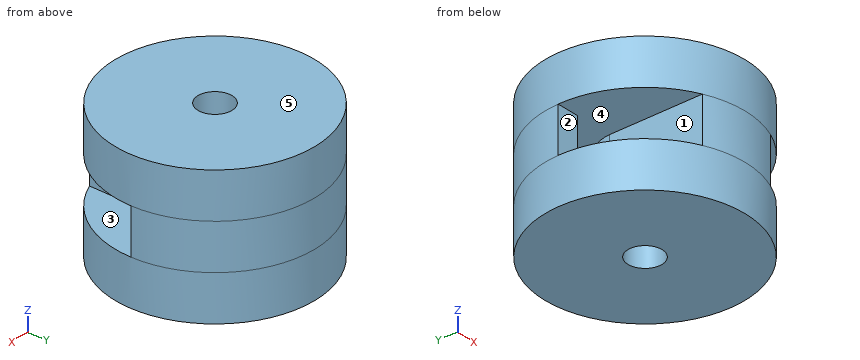
```python
from build123d import *

# Parameters (mm, degrees)
F0_R     = 11
F1_DEPTH = 5
F3_DEPTH = 5
F4_R     = 11
F5_DEPTH = 5
F6_R     = 1.875
F7_DEPTH = 25


with BuildPart() as f1:
    # F0 (on Top) → F1 (new body)
    with BuildSketch(Plane.XY):
        with Locations((-55.3302019835, -34.0237878263)):
            Circle(F0_R)
    extrude(amount=F1_DEPTH)

    # F2 (on face) → F3 (join)
    with BuildSketch(Plane.XY.offset(5)):
        with BuildLine():
            Line((-46.800726779, -33.8632795051), (-44.3313730877, -33.8632795051))
            ThreePointArc((-44.3313730877, -33.8632795051), (-55.3302019835, -23.0237878263), (-66.3290308792, -33.8632795051))
            Line((-66.3290308792, -33.8632795051), (-63.8596771879, -33.8632795051))
            ThreePointArc((-63.8596771879, -33.8632795051), (-55.3302019835, -25.9412589779), (-46.800726779, -33.8632795051))
        make_face()
        with BuildLine():
            ThreePointArc((-59.7163877129, -44.1114721367), (-55.3302019835, -45.0237878263), (-50.944016254, -44.1114721367))
            Line((-50.944016254, -44.1114721367), (-50.944016254, -34.1842961475))
            Line((-50.944016254, -34.1842961475), (-50.944016254, -33.8632795051))
            ThreePointArc((-50.944016254, -33.8632795051), (-55.3302019835, -29.6346662543), (-59.7163877129, -33.8632795051))
            Line((-59.7163877129, -33.8632795051), (-59.7163877129, -34.1842961475))
            Line((-59.7163877129, -34.1842961475), (-59.7163877129, -44.1114721367))
        make_face()
    extrude(amount=F3_DEPTH)

    # F4 (on face) → F5 (join)
    with BuildSketch(Plane.XY.offset(10)):
        with Locations((-55.3302019835, -34.0237878263)):
            Circle(F4_R)
    extrude(amount=F5_DEPTH)

    # F6 (on face) → F7 (cut)
    with BuildSketch(Plane.XY.offset(15)):
        with Locations((-55.3302019835, -34.0237878263)):
            Circle(F6_R)
    extrude(amount=-F7_DEPTH, mode=Mode.SUBTRACT)


solid = f1.part
```
Check sheet for the modelled part. Datum: model origin and axes. Units: mm. Face numbers are marked on the shaded views. A direction names the side the tool comes from. Round coordinates to 2 decimals unless told otherwise and drop trailing zeros. Order: outer loops, then holes, each group sorted by start corner. A loop starts at its lowest first (then second) coordinate and runs counter-clockwise, first axis right, second up. Notation, with made-up numbers: (39.25, -22) - (58.25, -22) arc R15 cw to (58.25, 0) - close; hole circle Ø3 at (6.5, 87.25). An arc over 180 degrees is marked (long way). Write item = value, one per line.
Q1. Go/stop test with flat-tipped pins: pin 1 (8 mm diameter, centred on x = -55.5, y = -41, fed in from -Z); pin 2 (4 mm diameter, centred on y = -41, z = 7.5, fed in from -X); pin 3 (2.5 mm diameter, centred on y = -37.5, z = 7, fed in from +X); pin 4 (5 mm diameter, centred on x = -62, z = 12, fed in from -Y). Record where each tip stops, or that it passes through.
Computed:
pin_1 = 0
pin_2 = -59.72
pin_3 = -50.94
pin_4 = -44.2
Q2. Section check A-A (y = -33). Record the boundary of the cut face in (x, z).
Computed:
outline = (-66.28, 0) - (-56.9, 0) - (-56.9, 15) - (-66.28, 15) - close; (-53.76, 0) - (-44.38, 0) - (-44.38, 15) - (-53.76, 15) - close; hole (-63.75, 5) - (-59.6, 5) - (-59.6, 10) - (-63.75, 10) - close; hole (-51.06, 5) - (-46.91, 5) - (-46.91, 10) - (-51.06, 10) - close
Q3. Section check C-C (z = 5.5). Record the boundary of the cut face in (x, y) (3 decimals), and give its area (3 significant figures).
Computed:
outline = (-66.329, -33.863) - (-63.86, -33.863) arc R8.553 cw to (-46.801, -33.863) - (-44.331, -33.863) arc R11 ccw to start; (-59.716, -44.111) arc R11 ccw to (-50.944, -44.111) - (-50.944, -33.863) arc R4.389 ccw to (-59.716, -33.863) - close; hole circle Ø3.75 at (-55.33, -34.024)
area = 196 mm^2
Q4. Thickness scan on line 1 along Z through (x, y) = (-60, -40.25); line 2 along X through (y, z) = (-33.5, 6) (3 decimals); line 3 along X through (y, z) = (-42.75, 5.5). Record the ranges inside material, lowest first.
Computed:
line_1 = 0 to 5, 10 to 15
line_2 = -66.318 to -63.825, -59.688 to -57.131, -53.53 to -50.972, -46.835 to -44.343
line_3 = -59.72 to -50.94
Q5. Tool access check on the marked faces 4 and 5. Record the directions out of +Z, -Z, +X, -X, +Y, -Y that give a thin tool (end or side, any length) a straight path to the whole face; none if there is none.
Computed:
face_4 = none
face_5 = +Z, +X, -X, +Y, -Y
Q6. Draft check along Y on the marked faces 1, 2 and 3. Enter one of: pulls with the +Y half, pulls with the -Y half, needs draft (parallel to the pull), parting line crosses it, or undercut.
Computed:
face_1 = needs draft
face_2 = pulls with the -Y half
face_3 = undercut
Q7. Section check D-D (y = -26.25). Record the boundary of the cut face in (x, z).
Computed:
outline = (-63.11, 0) - (-47.55, 0) - (-47.55, 15) - (-63.11, 15) - close; hole (-57.61, 5) - (-53.05, 5) - (-53.05, 10) - (-57.61, 10) - close
Q8. Section check B-B (x = -56.75). Record the boundary of the cut face in (y, z).
Computed:
outline = (-44.93, 0) - (-35.25, 0) - (-35.25, 15) - (-44.93, 15) - close; (-32.8, 0) - (-23.12, 0) - (-23.12, 15) - (-32.8, 15) - close; hole (-29.87, 5) - (-26.06, 5) - (-26.06, 10) - (-29.87, 10) - close
